Study the drawing (mm; zero at the part's minimum x, y, z) and answer. Round coordinates to 2 decimals unless told otherwise and drop trailing zeros. Write each loop counter-clockwise with the first axis right and the second up, starting at its lowest first coordinate (ties: lowest second). Pieces come first, ordered by that corner, then holes. Notation, with made-up numbers: (66.5, 21.25) -> (119.5, 21.25) arc R24 ccw to (119.5, 39.25) -> close; hole circle Ø4 at (24.25, 86.25). An arc over 180 degrees is marked (long way). Return JSON: item names as keys, results as strings.
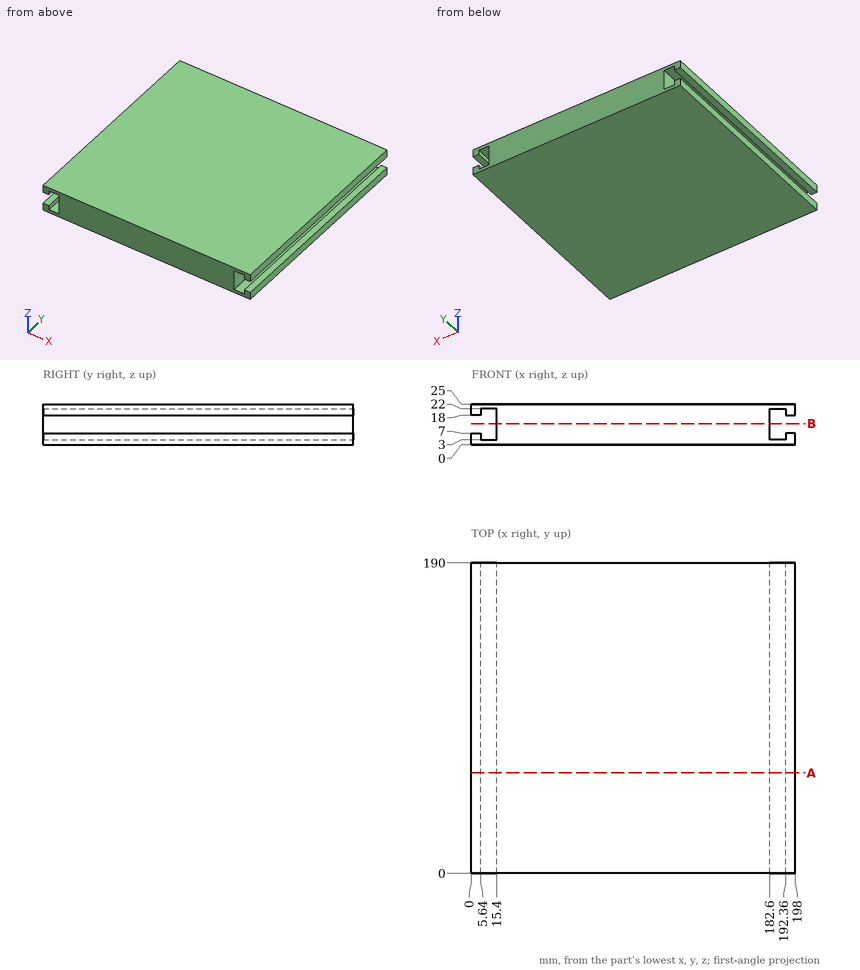
Item 1: Section B-B (z = 13) is taken. Give the vertices of the cut face in (x, y), then the cut area to 3 significant figures.
Worked answers:
{"outline": "(15.4, 0) -> (182.6, 0) -> (182.6, 190) -> (15.4, 190) -> close", "area": "31,800 mm2"}
Item 2: Straight lines are drawn through the part: L1, parallel to X at y = 117.5, z = 3.5; L2, parallel to Z at x = 186.5, y = 113; L3, parallel to X at y = 56.5, z = 16.25. For each, find the intervals that lie inside material, in ascending order. Write a range as [from, to].
Worked answers:
{"L1": "x = [0, 5.64], [15.4, 182.6], [192.36, 198]", "L2": "z = [0, 3], [22, 25]", "L3": "x = [15.4, 182.6]"}
Item 3: Section A-A (y = 61.5) is taken. Give the vertices of the cut face in (x, z), then the cut area to 4 significant figures.
Worked answers:
{"outline": "(0, 0) -> (198, 0) -> (198, 7) -> (192.36, 7) -> (192.36, 3) -> (182.6, 3) -> (182.6, 22) -> (192.36, 22) -> (192.36, 18) -> (198, 18) -> (198, 25) -> (0, 25) -> (0, 18) -> (5.64, 18) -> (5.64, 22) -> (15.4, 22) -> (15.4, 3) -> (5.64, 3) -> (5.64, 7) -> (0, 7) -> close", "area": "4,455 mm2"}
Item 4: A flat-ended cylindrical pin translates along its axis: pin 1 (1 mm diameter, centred on y = 42, z = 16, fed in from -X). Find the tip coordinate at first contact, or state that the pin passes through.
Worked answers:
{"pin 1": "stops at x = 15.4"}
